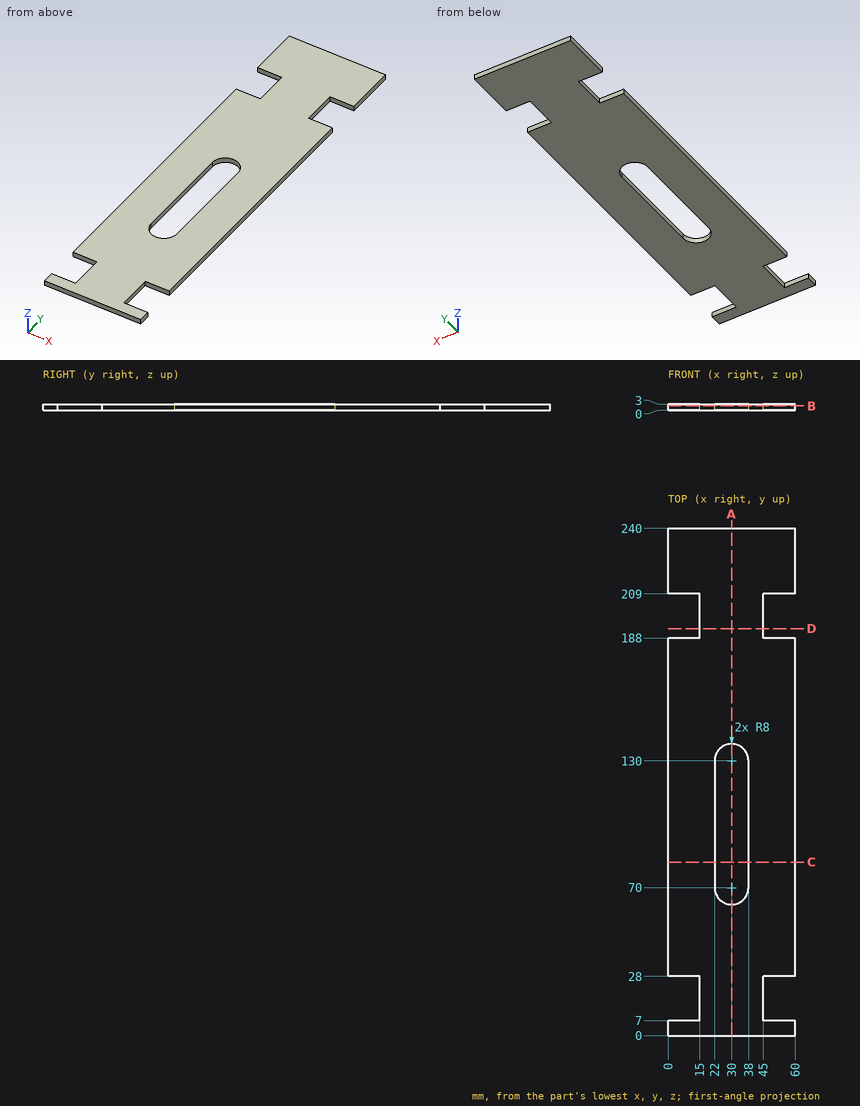
Study the drawing (mm; zero at the part's minimum x, y, z) and answer. Give positions to 0.01 mm unless a question says otherwise; leave off trailing zeros. Loops run counter-clockwise (first coordinate to the right, second up) from the corner with the lowest first, then second, coordinate; pieces in that order, holes last. Notation, with made-up numbers: (-40, 21) -> (-13, 21) arc R27 cw to (-13, 38) -> close; hole circle Ø8 at (80, 42.25). An arc over 180 degrees is marked (long way). Write item = value, one per line. Start each with the question number.
(1) Find section D-D on y = 192.5. Give the vertices of the cut face in (x, z), and give its area (3 significant figures).
(2) Find section A-A on x = 30. Give the vertices of the cut face in (y, z).
(3) Find the intervals of material crossed by probe 1 along Y at (x, z) = (5, 0.5); probe 2 along X at (y, z) = (112, 0.4); probe 3 along X at (y, z) = (207.5, 2.55), in increasing order. Write a range as from..to.
(4) Find section C-C on y = 82. Give the vertices of the cut face in (x, z), and give its area (3 significant figures).
(5) Given pin 1 Ø1.5 at (y, z) = (198.5, 1) entering from +X, flat-ended and moving along its own axis, determine where the tip first touches the part or whether it passes through.
(6) Find section B-B on z = 2.15. Give the vertices of the cut face in (x, y).
From the geometry:
q1.outline = (15, 0) -> (45, 0) -> (45, 3) -> (15, 3) -> close
q1.area = 90.0 mm^2
q2.outline = (0, 0) -> (62, 0) -> (62, 3) -> (0, 3) -> close; (138, 0) -> (240, 0) -> (240, 3) -> (138, 3) -> close
q3.probe_1 = 0..7, 28..188, 209..240
q3.probe_2 = 0..22, 38..60
q3.probe_3 = 15..45
q4.outline = (0, 0) -> (22, 0) -> (22, 3) -> (0, 3) -> close; (38, 0) -> (60, 0) -> (60, 3) -> (38, 3) -> close
q4.area = 132 mm^2
q5.pin_1 = 45
q6.outline = (0, 0) -> (60, 0) -> (60, 7) -> (45, 7) -> (45, 28) -> (60, 28) -> (60, 188) -> (45, 188) -> (45, 209) -> (60, 209) -> (60, 240) -> (0, 240) -> (0, 209) -> (15, 209) -> (15, 188) -> (0, 188) -> (0, 28) -> (15, 28) -> (15, 7) -> (0, 7) -> close; hole (22, 70) arc R8 ccw to (38, 70) -> (38, 130) arc R8 ccw to (22, 130) -> close
